Could you check a few things on this model? Use its own coordinates, in mm. Round coordinates to 2 decimals unless told otherwise and drop trailing zeros. Loops run counter-clockwise (first coordinate to the right, second up) from the corner with the lowest first, then second, coordinate; pieces in that order, holes last. Notation, with made-up numbers: (23, 33) -> (67, 33) arc R16 ccw to (67, 47) -> close; hole circle Ø4 at (67.25, -25.75). An arc over 180 degrees is marked (long way). One line per item, written item: value.
from build123d import *

# Parameters (mm, degrees)
F0_W     = 90
F0_H     = 115
F0_R     = 1.6
F0_R_2   = 1.1
F1_DEPTH = 2
F2_SIZE  = 0.2


with BuildPart() as f1:
    # F0 (on Front) → F1 (new body)
    with BuildSketch(Plane.XZ):
        Rectangle(F0_W, F0_H)
        with Locations((-7.5, -52.5)):
            Circle(F0_R, mode=Mode.SUBTRACT)
        with Locations((-38, -7.7)):
            Circle(F0_R, mode=Mode.SUBTRACT)
        with Locations((28, -4.5)):
            Circle(F0_R, mode=Mode.SUBTRACT)
        with Locations((-28, 15.052562)):
            Circle(F0_R_2, mode=Mode.SUBTRACT)
        with Locations((-38, 45.052562)):
            Circle(F0_R_2, mode=Mode.SUBTRACT)
        with Locations((-37.5, 52.5)):
            Circle(F0_R, mode=Mode.SUBTRACT)
        with Locations((-7.5, 30.052562)):
            Circle(F0_R, mode=Mode.SUBTRACT)
        with Locations((-18, 45.052562)):
            Circle(F0_R_2, mode=Mode.SUBTRACT)
        with Locations((-7.5, 45.052562)):
            Circle(F0_R, mode=Mode.SUBTRACT)
        with Locations((37.5, 7.5)):
            Circle(F0_R, mode=Mode.SUBTRACT)
        with Locations((7.5, 30.052562)):
            Circle(F0_R, mode=Mode.SUBTRACT)
        with Locations((7.5, 45.052562)):
            Circle(F0_R, mode=Mode.SUBTRACT)
        with Locations((22.5, 30.052562)):
            Circle(F0_R_2, mode=Mode.SUBTRACT)
        with Locations((37.5, 30.052562)):
            Circle(F0_R_2, mode=Mode.SUBTRACT)
        with Locations((22.5, 45.052562)):
            Circle(F0_R_2, mode=Mode.SUBTRACT)
        with Locations((37.5, 45.052562)):
            Circle(F0_R_2, mode=Mode.SUBTRACT)
        with Locations((37.5, 52.5)):
            Circle(F0_R, mode=Mode.SUBTRACT)
    extrude(amount=F1_DEPTH)

    # F2
    f2_edges = [f1.edges().sort_by_distance(p)[0] for p in [
        (45, -2, 0),
        (0, -2, -57.5),
        (45, 0, 0),
        (0, 0, -57.5),
        (45, -1, -57.5),
        (-45, -1, -57.5),
        (-45, -2, 0),
        (-45, 0, 0),
        (0, 0, 57.5),
        (-9.1, 0, -52.5),
        (-39.6, 0, -7.7),
        (26.4, 0, -4.5),
        (-29.1, 0, 15.052562),
        (-39.1, 0, 45.052562),
        (-39.1, 0, 52.5),
        (-9.1, 0, 30.052562),
        (-19.1, 0, 45.052562),
        (-9.1, 0, 45.052562),
        (35.9, 0, 7.5),
        (5.9, 0, 30.052562),
        (5.9, 0, 45.052562),
        (21.4, 0, 30.052562),
        (36.4, 0, 30.052562),
        (21.4, 0, 45.052562),
        (36.4, 0, 45.052562),
        (35.9, 0, 52.5),
        (0, -2, 57.5),
        (45, -1, 57.5),
        (-45, -1, 57.5),
    ]]
    chamfer(f2_edges, length=F2_SIZE)


solid = f1.part
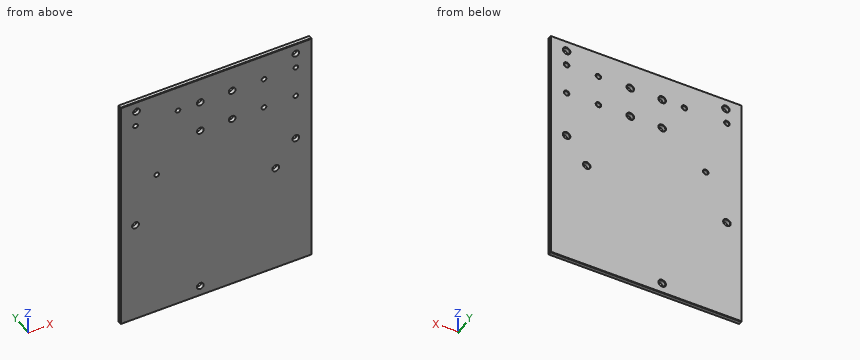
(1) If I drill on L1, parallel to Z at x = 7.5, y = -0.65; L2, parallel to X at y = -1.15, z = 51.5; L3, parallel to Z at x = 29, y = -0.05, over which ranges is the centre line in solid material (lowest first)?
Recorded:
L1: -57.5 to 28.45, 31.65 to 43.45, 46.65 to 57.5
L2: -45 to -38.75, -36.25 to 36.25, 38.75 to 45
L3: -57.35 to -5.94, -3.06 to 57.35
(2) If we section it at A-A, the plane z = -4.5: Please give me the cut outline in (x, y), then the cut area to 3 significant figures.
Recorded:
outline: (-45, -1.8) -> (-44.8, -2) -> (26.4, -2) -> (26.4, -0.2) -> (26.2, 0) -> (-44.8, 0) -> (-45, -0.2) -> close; (29.6, -2) -> (44.8, -2) -> (45, -1.8) -> (45, -0.2) -> (44.8, 0) -> (29.8, 0) -> (29.6, -0.2) -> close
area: 173 mm²
(3) If we section it at C-C, the plane x = -7.5: Please give me the cut outline in (y, z).
Recorded:
outline: (-2, -57.3) -> (-1.8, -57.5) -> (-0.2, -57.5) -> (0, -57.3) -> (0, -54.3) -> (-0.2, -54.1) -> (-2, -54.1) -> close; (-2, -50.9) -> (-0.2, -50.9) -> (0, -50.7) -> (0, 28.25) -> (-0.2, 28.45) -> (-2, 28.45) -> close; (-2, 31.65) -> (-0.2, 31.65) -> (0, 31.85) -> (0, 43.25) -> (-0.2, 43.45) -> (-2, 43.45) -> close; (-2, 46.65) -> (-0.2, 46.65) -> (0, 46.85) -> (0, 57.3) -> (-0.2, 57.5) -> (-1.8, 57.5) -> (-2, 57.3) -> close
(4) If we section it at B-B, the plane x = 28: Please give me the cut outline in (y, z), then the cut area to 3 significant figures.
Recorded:
outline: (-2, -57.3) -> (-1.8, -57.5) -> (-0.2, -57.5) -> (0, -57.3) -> (0, -6.3) -> (-0.2, -6.1) -> (-2, -6.1) -> close; (-2, -2.9) -> (-0.2, -2.9) -> (0, -2.7) -> (0, 57.3) -> (-0.2, 57.5) -> (-1.8, 57.5) -> (-2, 57.3) -> close
area: 223 mm²
(5) I'm going to push flat-ended pins straight in: pin 1 Ø3.5 at (x, z) = (-7.5, 45.05) entering from +Y; pin 2 Ø3 at (x, z) = (-7.5, 30.05) entering from -Y. Where does each tip first touch, or does it pass through?
Recorded:
pin 1: y = -0.05
pin 2: through
